```python
from build123d import *

# Parameters (mm, degrees)
SKETCH4_R           = 2.5
BOSS_EXTRUDE2_DEPTH = 7.5
CUT_EXTRUDE1_DEPTH  = 35.126684354
SKETCH4_4_R         = 2.5
BOSS_EXTRUDE4_DEPTH = 0.5
BOSS_EXTRUDE5_START = 7
SKETCH4_5_R         = 2.5
BOSS_EXTRUDE5_DEPTH = 0.5


with BuildPart() as part:
    # Sketch4 → Boss-Extrude2 (new body)
    with BuildSketch(Plane(origin=(0, 0, 0), x_dir=(0, 0, -1), z_dir=(1, 0, 0))):
        with BuildLine():
            Line((28.269557121, 8.217760269), (30.746429201, 9.303054261))
            ThreePointArc((30.746429201, 9.303054261), (31.323725134, 10.424611444), (30.343861951, 11.218984941))
            ThreePointArc((30.343861951, 11.218984941), (13.830620655, 9.141504786), (-1.66846042, 3.076725504))
            ThreePointArc((-1.66846042, 3.076725504), (-2.603150363, -2.33957436), (2.881836513, -1.986207016))
            ThreePointArc((2.881836513, -1.986207016), (13.025423778, 6.31803392), (26.035044154, 7.931278408))
            ThreePointArc((26.035044154, 7.931278408), (27.172885501, 7.913960675), (28.269557121, 8.217760269))
        make_face()
        Circle(SKETCH4_R, mode=Mode.SUBTRACT)
    extrude(amount=BOSS_EXTRUDE2_DEPTH)

    # Sketch5 → Cut-Extrude1 (cut, through all)
    with BuildSketch(Plane(origin=(0, 0, 0), x_dir=(1, 0, 0), z_dir=(0, 1, 0))):
        with BuildLine():
            Line((1.5, 2.5), (1.5, -2.5))
            ThreePointArc((1.5, -2.5), (3.75, -4.75), (6, -2.5))
            Line((6, -2.5), (6, 2.5))
            ThreePointArc((6, 2.5), (3.75, 4.75), (1.5, 2.5))
        make_face()
    extrude(amount=-CUT_EXTRUDE1_DEPTH, mode=Mode.SUBTRACT)

    # Sketch4<4> → Boss-Extrude4 (add)
    with BuildSketch(Plane(origin=(0, 0, 0), x_dir=(0, 0, -1), z_dir=(1, 0, 0))):
        Circle(SKETCH4_4_R)
    extrude(amount=BOSS_EXTRUDE4_DEPTH)

    # Sketch4<5> → Boss-Extrude5 (add)
    with BuildSketch(Plane(origin=(0, 0, 0), x_dir=(0, 0, -1), z_dir=(1, 0, 0)).offset(BOSS_EXTRUDE5_START)):
        Circle(SKETCH4_5_R)
    extrude(amount=BOSS_EXTRUDE5_DEPTH)


solid = part.part
```
Geometry: final body of the model. Coordinates: model frame, mm. A direction names the side the tool comes from. Round coordinates to 2 decimals unless told otherwise and drop trailing zeros. Order: outer loops, then holes, each group sorted by start corner. A loop starts at its lowest first (then second) coordinate and runs counter-clockwise, first axis right, second up. Notation, with made-up numbers: (29.5, -22.75) - (39.5, -22.75) arc R32 cw to (39.5, 8.25) - close; hole circle Ø4 at (23.5, -5). An arc over 180 degrees is marked (long way). Use CSV: the item, a comma, the result in double quotes. Start each with the question number.
Q1. Access query for faces 1 (the face through (0.5, 0, 0)), 2 (the face through (3.698, 0.335, 3.484)), 3 (the face through (1.594, -0.663, -3.142)). Directions: +Z, -Z, +X, -X, +Y, -Y. A direction counts if a zero-diameter tool reaches every point of the face in a straight line with its end or side. Return the directions, or none.
Q2. Section query D-D (y = 4). Return loops of the section in (x, z).
Q3. First-contact query: pin 1 (1.5 mm diameter, centred on x = 5, z = -3, fed in from -Y); pin 2 (2 mm diameter, centred on x = 2, z = -13, fed in from +Y); pin 3 (2 mm diameter, centred on y = 6.5, z = -2, fed in from -X); pin 4 (4 mm diameter, centred on x = 3, y = 7, fed in from +Z). Flat tips, straight axial feed; report the tip coordinate or a pass-through.
Q4. Material intervals for line 1 along Z through (x, y) = (3.25, 1.75); line 2 along Y through (x, z) = (3.25, 0); line 3 along Z through (x, y) = (6.5, 2.75), sorted ascending. Write a range as from..to.
Q5. Section query C-C (x = 4). Return loops of the section in (y, z).
Q6. Mould query, pull axis Z, two halves, no side actions, for faces 4 (the face through (3.698, 8.753, -29.491)), 5 (the face through (7.5, 5, -10)), 6 (the face through (3.698, 7.912, -27.157)). Classes: +Z half, -Z half, draft (parallel to the pull), parting line (faces both ways), or undercut.
Q7. Section query B-B (z = 0). Return loops of the section in (x, y), and give its area (3 significant figures).
Q8. Section query A-A (y = 1.25). Return loops of the section in (x, z), and give its area (3 significant figures).
Result set:
1,face 1,"none"
1,face 2,"+X, -X"
1,face 3,"-Y"
2,outline,"(0, -8.84) - (7.5, -8.84) - (7.5, -0.1) - (0, -0.1) - close"
3,pin 1,"stops at y = 0"
3,pin 2,"stops at y = 9.18"
3,pin 3,"passes through"
3,pin 4,"stops at z = -2.16"
4,line 1,"z = -6.08..-1.79, 1.79..3.03"
4,line 2,"y = 2.5..3.95"
4,line 3,"z = -7.2..2.17"
5,outline,"(0, -4.41) arc R23.61 cw to (7.93, -26.04) arc R4 ccw to (8.22, -28.27) - (9.3, -30.75) arc R1 ccw to (11.22, -30.34) arc R67.33 ccw to (3.08, 1.67) arc R3.5 ccw to (0, 3.5) - (0, 2.5) arc R2.5 cw to (0, -2.5) - close"
6,face 4,"-Z half"
6,face 5,"draft"
6,face 6,"undercut"
7,outline,"(0, -3.5) - (1.5, -3.5) - (1.5, -2.5) - (0.5, -2.5) - (0.5, 2.5) - (7, 2.5) - (7, -2.5) - (6, -2.5) - (6, -3.5) - (7.5, -3.5) - (7.5, 3.95) - (0, 3.95) - close"
7,area,"18.9 mm2"
8,outline,"(0, -5.57) - (7.5, -5.57) - (7.5, 3.27) - (0, 3.27) - close; hole (0.5, -2.17) - (7, -2.17) - (7, 2.17) - (0.5, 2.17) - close"
8,area,"38.1 mm2"
